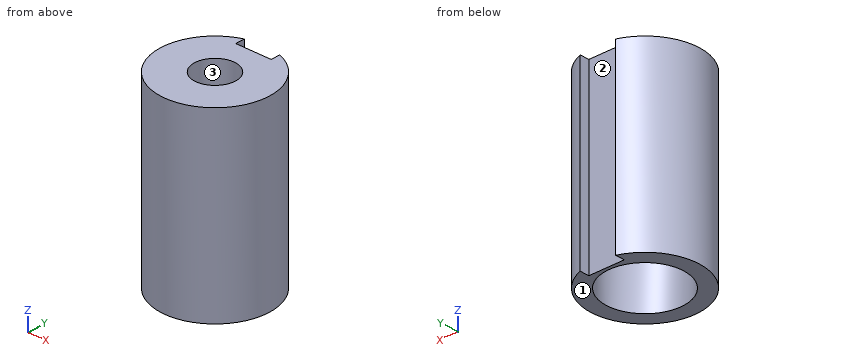
```python
from build123d import *

# Parameters (mm, degrees)
ESQUISSE1_R             = 11.925
BOSS_EXTRU_1_DEPTH      = 40.1
ESQUISSE2_R             = 8.5
ENL_V_MAT_EXTRU_1_DEPTH = 9.77
ENL_V_MAT_EXTRU_2_DEPTH = 15.5
ESQUISSE5_R             = 4.5
ENL_V_MAT_EXTRU_3_DEPTH = 41.1
ENL_V_MAT_EXTRU_5_DEPTH = 41.1


with BuildPart() as part:
    # Esquisse1 → Boss.-Extru.1 (new body)
    with BuildSketch(Plane.XY):
        Circle(ESQUISSE1_R)
    extrude(amount=BOSS_EXTRU_1_DEPTH)

    # Esquisse2 → Enlèv. mat.-Extru.1 (cut)
    with BuildSketch(Plane.XY):
        Circle(ESQUISSE2_R)
    extrude(amount=ENL_V_MAT_EXTRU_1_DEPTH, mode=Mode.SUBTRACT)

    # Esquisse4 → Enlèv. mat.-Extru.2 (cut)
    with BuildSketch(Plane(origin=(0, 0, 9.77), x_dir=(-1, 0, 0), z_dir=(0, 0, -1))):
        with BuildLine():
            Line((-6.498055974, 5.479531783), (6.411422693, 5.580650415))
            ThreePointArc((6.411422693, 5.580650415), (0.066577592, -8.499739256), (-6.498055974, 5.479531783))
        make_face()
    extrude(amount=-ENL_V_MAT_EXTRU_2_DEPTH, mode=Mode.SUBTRACT)

    # Esquisse5 → Enlèv. mat.-Extru.3 (cut, through all)
    with BuildSketch(Plane.XY.offset(40.1)):
        Circle(ESQUISSE5_R)
    extrude(amount=-ENL_V_MAT_EXTRU_3_DEPTH, mode=Mode.SUBTRACT)

    # Esquisse6 → Enlèv. mat.-Extru.5 (cut, through all)
    with BuildSketch(Plane.XY.offset(40.1)):
        with BuildLine():
            Line((-3.9, 11.269233559), (-3.9, 9.199599168))
            Line((-3.9, 9.199599168), (3.9, 9.199599168))
            Line((3.9, 9.199599168), (3.9, 11.269233559))
            ThreePointArc((3.9, 11.269233559), (0, 11.925), (-3.9, 11.269233559))
        make_face()
    extrude(amount=-ENL_V_MAT_EXTRU_5_DEPTH, mode=Mode.SUBTRACT)


solid = part.part
```
CAD build for the part. Positions are in the model's coordinates, mm. Face numbers are marked on the shaded views. Coordinates: 2 decimals unless noted, no trailing zeros. Order: outer loops, then holes, each group sorted by start corner. A loop starts at its lowest first (then second) coordinate and runs counter-clockwise, first axis right, second up.
(1) Drill centre lines: L1, parallel to X at y = 0, z = 20 (3 decimals); L2, parallel to Y at x = 0, z = 34.5 (3 decimals); L3, parallel to Z at x = 8.25, y = 0.75. Where is each one in solid material? Low to high.
Solution:
L1: x = -11.925 to -8.5, 8.5 to 11.925
L2: y = -11.925 to -4.5, 4.5 to 9.2
L3: z = 25.27 to 40.1
(2) Saw through at C-C, the plane x = 1. Write the cut outline in (y, z).
Solution:
outline: (-11.88, 0) - (-8.44, 0) - (-8.44, 25.27) - (-4.39, 25.27) - (-4.39, 40.1) - (-11.88, 40.1) - close; (4.39, 25.27) - (5.52, 25.27) - (5.52, 9.77) - (8.44, 9.77) - (8.44, 0) - (9.2, 0) - (9.2, 40.1) - (4.39, 40.1) - close
(3) Pin check, flat tips, straight feed: pin 1 Ø7 at (x, y) = (2.5, -1) entering from -Z; pin 2 Ø4 at (x, z) = (-6, 20) entering from -Y; pin 3 Ø0.6 at (y, z) = (10.5, 25) entering from -X; pin 4 Ø8 at (x, y) = (0, 0) entering from +Z. Stop position of each tip, or through.
Solution:
pin 1: stops at z = 25.27
pin 2: stops at y = -11.23
pin 3: stops at x = -6.18
pin 4: passes through
(4) Saw through at D-D, the plane y = -3.25. Write the cut outline in (x, z), and give its area (3 significant figures).
Solution:
outline: (-11.47, 0) - (-7.85, 0) - (-7.85, 25.27) - (-3.11, 25.27) - (-3.11, 40.1) - (-11.47, 40.1) - close; (3.11, 25.27) - (7.85, 25.27) - (7.85, 0) - (11.47, 0) - (11.47, 40.1) - (3.11, 40.1) - close
area: 431 mm2
(5) Saw through at B-B, the plane z = 9. Write the cut outline in (x, y) (3 decimals).
Solution:
outline: (-3.9, 9.2) - (-3.9, 11.269) arc R11.925 ccw (long way) to (3.9, 11.269) - (3.9, 9.2) - close; hole circle Ø17 at (0, 0)
(6) Saw through at A-A, the plane y = 0. Write the cut outline in (x, z) (3 decimals).
Solution:
outline: (-11.925, 0) - (-8.5, 0) - (-8.5, 25.27) - (-4.5, 25.27) - (-4.5, 40.1) - (-11.925, 40.1) - close; (4.5, 25.27) - (8.5, 25.27) - (8.5, 0) - (11.925, 0) - (11.925, 40.1) - (4.5, 40.1) - close
(7) Mould opens along Y. For the marked faces 1, 2 and 3 say: released by +Y, released by -Y, zero draft, split by the parting line, or undercut.
Solution:
face 1: zero draft
face 2: released by +Y
face 3: undercut
